Here's how the part is built. I have some questions about the finished solid (model axes, mm). Face numbers are marked on the shaded views. A direction names the side the tool comes from. Round coordinates to 2 decimals unless told otherwise and drop trailing zeros. Write each loop counter-clockwise with the first axis right and the second up, starting at its lowest first coordinate (ties: lowest second). Pieces come first, ordered by that corner, then holes. Notation, with made-up numbers: (-19, 71.25) - (28, 71.25) arc R26 ccw to (28, 89.25) - close; hole circle Ø3 at (3, 46). An arc over 180 degrees is marked (long way). Return JSON: item names as keys, results as strings. Group by question number.
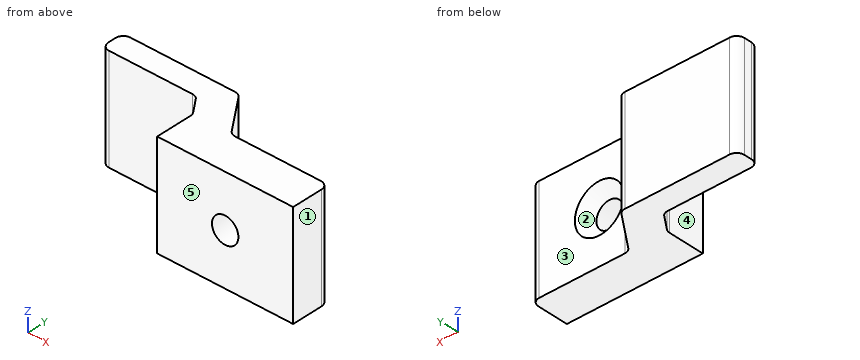
```python
from build123d import *

# Parameters (mm, degrees)
EXTRUDE_442_DEPTH          = 13.5
FILLET_1_R                 = 1
HOLE_WIZARD_M3_D           = 3.4
HOLE_WIZARD_M3_CSINK_D     = 6.3
HOLE_WIZARD_M3_CSINK_ANGLE = 90


with BuildPart() as part:
    # Эскиз1 → Extrude 442 (new body)
    with BuildSketch(Plane.XY):
        Polygon((8.75, 0), (-8.75, 0), (-8.75, 5), (-10.564997351, 7.5), (-22.8, 7.5), (-22.8, 10.5), (-7.8, 10.5), (-3.807005828, 5), (8.75, 5), align=None)
    extrude(amount=EXTRUDE_442_DEPTH)

    # Скругление1
    fillet_1_edges = [part.edges().sort_by_distance(p)[0] for p in [
        (-8.75, 5, 6.75),
        (-10.564997351, 7.5, 6.75),
        (-22.8, 7.5, 6.75),
        (-22.8, 10.5, 6.75),
        (-7.8, 10.5, 6.75),
        (-3.807005828, 5, 6.75),
        (8.75, 5, 6.75),
    ]]
    fillet(fillet_1_edges, radius=FILLET_1_R)

    # Крепление-M3 (through all)
    with Locations(Plane(origin=(0, 5, 0), x_dir=(1, 0, 0), z_dir=(0, 1, 0))):
        with Locations((0, -6.75)):
            CounterSinkHole(HOLE_WIZARD_M3_D / 2, HOLE_WIZARD_M3_CSINK_D / 2, counter_sink_angle=HOLE_WIZARD_M3_CSINK_ANGLE)


solid = part.part
```
1) If we mould it in two halves opening along X, with no side actions, what happens to the marked faces 1, 2 and 3? For each: released by +X, released by -X, zero draft, split by the parting line, or undercut.
2) Imagine slicing it at D-D (z = 10.5). Please give me the cut outline in (x, y).
3) Imagine slicing it at B-B (x = 0). Please give me the cut outline in (y, z), plus the area to 3 significant figures.
4) I need wall thicknesses on line 1 along Z through (x, y) = (0, 1.9); line 2 along X through (y, z) = (1.7, 6.75); line 3 along X through (y, z) = (2, 2.25). Which ranges of each line are inside material? Lowest first, please.
5) Will these pins go through, and if not, where does the flat tip stop? pin 1 Ø5 at (y, z) = (3, 7) entering from -X; pin 2 Ø1 at (y, z) = (8, 2) entering from +X; pin 3 Ø3 at (x, z) = (-17.5, 9) entering from -Y.
6) Imagine slicing it at A-A (z = 6.75). Please give me the cut outline in (x, y), plus the area to 3 significant figures.
7) For the marked faces 4 and 5, which set-ups out of +Z, -Z, +X, -X, +Y, -Y let a thin tool reach every point of the face, with its end or its side?
8) Imagine slicing it at C-C (y = 1.75). Please give me the cut outline in (x, z).
Results found:
{
 "1": {"face 1": "released by +X", "face 2": "undercut", "face 3": "zero draft"},
 "2": {"outline": "(-22.8, 8.5) arc R1 ccw to (-21.8, 7.5) - (-11.07, 7.5) arc R1 cw to (-10.27, 7.09) - (-8.94, 5.26) arc R1 cw to (-8.75, 4.68) - (-8.75, 0) - (8.75, 0) - (8.75, 4) arc R1 ccw to (7.75, 5) - (-3.3, 5) arc R1 cw to (-4.11, 5.41) - (-7.5, 10.09) arc R1 ccw to (-8.31, 10.5) - (-21.8, 10.5) arc R1 ccw to (-22.8, 9.5) - close"},
 "3": {"outline": "(0, 0) - (5, 0) - (5, 3.6) - (3.55, 5.05) - (0, 5.05) - close; (0, 8.45) - (3.55, 8.45) - (5, 9.9) - (5, 13.5) - (0, 13.5) - close", "area": "48.4 mm²"},
 "4": {"line 1": "z = 0 to 5.05, 8.45 to 13.5", "line 2": "x = -8.75 to -1.7, 1.7 to 8.75", "line 3": "x = -8.75 to 8.75"},
 "5": {"pin 1": "stops at x = -9.11", "pin 2": "stops at x = -5.62", "pin 3": "stops at y = 7.5"},
 "6": {"outline": "(-22.8, 8.5) arc R1 ccw to (-21.8, 7.5) - (-11.07, 7.5) arc R1 cw to (-10.27, 7.09) - (-8.94, 5.26) arc R1 cw to (-8.75, 4.68) - (-8.75, 0) - (-1.7, 0) - (-1.7, 3.55) - (-3.15, 5) - (-3.3, 5) arc R1 cw to (-4.11, 5.41) - (-7.5, 10.09) arc R1 ccw to (-8.31, 10.5) - (-21.8, 10.5) arc R1 ccw to (-22.8, 9.5) - close; (1.7, 0) - (8.75, 0) - (8.75, 4) arc R1 ccw to (7.75, 5) - (3.15, 5) - (1.7, 3.55) - close", "area": "128 mm²"},
 "7": {"face 4": "+Z, -Z, -X, -Y", "face 5": "+Z, -Z, +X, -X, -Y"},
 "8": {"outline": "(-8.75, 0) - (8.75, 0) - (8.75, 13.5) - (-8.75, 13.5) - close; hole circle Ø3.4 at (0, 6.75)"}
}
